For this review, take the finished solid that the model builds, in its own axes (mm). Give positions to 0.01 mm unless a question says otherwise; leave off trailing zeros. Answer as CSV lines item,"result".
```python
from build123d import *


# Not quite as in the source:
# - a feature names something its author has since deleted; it is built from what else it names


with BuildPart() as f1:
    # F0 (on Front) → F1 (revolve)
    with BuildSketch(Plane.XZ):
        with BuildLine():
            Line((628.65, 0), (615.95, 0))
            Line((615.95, 0), (615.95, -12.7))
            Line((615.95, -12.7), (637.4086206897, -21.8965517241))
            ThreePointArc((637.4086206897, -21.8965517241), (630.9208650644, -11.7916539742), (628.65, 0))
        make_face()
        with BuildLine():
            Line((615.95, 12.7), (615.95, 0))
            Line((615.95, 0), (628.65, 0))
            ThreePointArc((628.65, 0), (630.9208650644, 11.7916539742), (637.4086206897, 21.8965517241))
            Line((637.4086206897, 21.8965517241), (615.95, 12.7))
        make_face()
        with BuildLine():
            ThreePointArc((637.4086206897, 21.8965517241), (630.9208650644, 11.7916539742), (628.65, 0))
            ThreePointArc((628.65, 0), (630.9208650644, -11.7916539742), (637.4086206897, -21.8965517241))
            Line((637.4086206897, -21.8965517241), (660.4, -31.75))
            ThreePointArc((660.4, -31.75), (682.7606574143, -22.5402639736), (692.1489839837, -0.254))
            Line((692.1489839837, -0.254), (689.61, -0.254))
            Line((689.61, -0.254), (689.61, 0))
            Line((689.61, 0), (689.61, 0.254))
            Line((689.61, 0.254), (692.1489839837, 0.254))
            ThreePointArc((692.1489839837, 0.254), (682.7606574143, 22.5402639736), (660.4, 31.75))
            Line((660.4, 31.75), (637.4086206897, 21.8965517241))
        make_face()
        with BuildLine():
            ThreePointArc((660.4, 31.75), (647.8930622701, 29.1828547031), (637.4086206897, 21.8965517241))
            Line((637.4086206897, 21.8965517241), (660.4, 31.75))
        make_face()
        with BuildLine():
            Line((660.4, -31.75), (637.4086206897, -21.8965517241))
            ThreePointArc((637.4086206897, -21.8965517241), (647.8930622701, -29.1828547031), (660.4, -31.75))
        make_face()
    revolve(axis=Axis((0, 0, 41.6052), (0, 0, 1)))


solid = f1.part
```
Q1. To check wall thickness, follow probe 1 along Y at (x, z) = (0, 3); probe 2 along Y at (x, z) = (0, 1.75); probe 3 along X at (y, z) = (158, 18). State the ranges of each line that lie inside material, in increasing order. Write a range as [from, to].
Answer block:
probe 1,"y = [-692.01, -615.95], [615.95, 692.01]"
probe 2,"y = [-692.1, -615.95], [615.95, 692.1]"
probe 3,"x = [-668.13, -608.13], [608.13, 668.13]"
Q2. Clearance check with flat-ended pins moving along their axes: pin 1 (8 mm diameter, centred on x = 88, z = 14.5, fed in from +Y); pin 2 (4 mm diameter, centred on x = -358, z = -15.5, fed in from +Y); pin 3 (1 mm diameter, centred on x = -110.5, z = 7.5, fed in from -Y). State where each tip first meets the part, or that it passes through.
Answer block:
pin 1,"stops at y = 684.82"
pin 2,"stops at y = 589.38"
pin 3,"stops at y = -682.51"
Q3. Draft analysis for pull direction X (two halves, no side actions). For faces 1 (the conical face through (588.787, 185.418, -13.275)), 2 (the cylindrical face through (-508.27, 466.07, 0)), state which applies: released by +X, released by -X, zero draft, split by the parting line, or undercut.
Answer block:
face 1,"undercut"
face 2,"split by the parting line"
